```python
from build123d import *

# Parameters (mm, degrees)
SKETCH1_W           = 500
SKETCH1_H           = 50
BOSS_EXTRUDE1_DEPTH = 25
SKETCH2_R           = 10
CUT_EXTRUDE1_DEPTH  = 257.173769149
SKETCH4_R           = 25
BOSS_EXTRUDE2_DEPTH = 200
BOSS_EXTRUDE3_START = 200
SKETCH5_R           = 25
BOSS_EXTRUDE3_DEPTH = 200


with BuildPart() as part:
    # Sketch1 → Boss-Extrude1 (new, symmetric)
    with BuildSketch(Plane(origin=(0, 0, 0), x_dir=(1, 0, 0), z_dir=(0, 1, 0))):
        Rectangle(SKETCH1_W, SKETCH1_H)
    extrude(amount=BOSS_EXTRUDE1_DEPTH, both=True)

    # Sketch2 → Cut-Extrude1 (cut, through all)
    with BuildSketch(Plane(origin=(0, 25, 0), x_dir=(1, 0, 0), z_dir=(0, 1, 0))):
        with Locations(Location((200, 0, 0), (0, 0, 270))):
            Circle(SKETCH2_R)
        with Locations(Location((-200, 0, 0), (0, 0, 90))):
            Circle(SKETCH2_R)
    extrude(amount=-CUT_EXTRUDE1_DEPTH, mode=Mode.SUBTRACT)

    # Sketch4 → Boss-Extrude2 (add)
    with BuildSketch(Plane(origin=(250, 0, 0), x_dir=(0, 0, -1), z_dir=(1, 0, 0))):
        Circle(SKETCH4_R)
    extrude(amount=BOSS_EXTRUDE2_DEPTH)

    # Sketch5 → Boss-Extrude3 (add)
    with BuildSketch(Plane.ZY.offset(250).offset(BOSS_EXTRUDE3_START)):
        with Locations(Location((0, 0, 0), (0, 0, 180))):
            Circle(SKETCH5_R)
    extrude(amount=-BOSS_EXTRUDE3_DEPTH)


solid = part.part
```
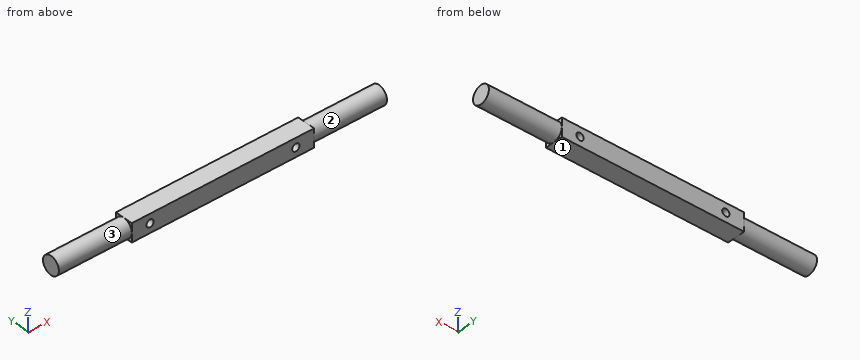
The model under review builds one solid part; all positions refer to its coordinate system, in mm. Face numbers are marked on the shaded views. A direction names the side the tool comes from. Coordinates: 2 decimals unless noted, no trailing zeros. Write each loop counter-clockwise with the first axis right and the second up, starting at its lowest first coordinate (ties: lowest second). Pieces come first, ordered by that corner, then holes. Notation, with made-up numbers: (66.25, 72) -> (70.25, 72) arc R28 cw to (70.25, 103) -> close; hole circle Ø4 at (68, 36). An arc over 180 degrees is marked (long way). One line per item, written item: value. Start each with the question number.
Q1. To check wall thickness, follow probe 1 along X at (y, z) = (2.5, 0); probe 2 along X at (y, z) = (2, 9); probe 3 along Z at (x, y) = (-200, 4). State the ranges of each line that lie inside material, in increasing order.
Q2. Add section A-A, the plane x = 200. Give the boundary of the cut face in (y, z).
Q3. Clearance check with flat-ended pins moving along their axes: P1, Ø12, axis at x = -284, z = -19, coming from the -Y side; P2, Ø3, axis at x = 260.5, y = -7.5, coming from the +Z side; P3, Ø5, axis at x = -310.5, z = 11, coming from the -Y side. State where each tip first meets the part, or that it passes through.
Q4. For the marked faces 1, 2 and 3, list the 3-axis set-ups (+Z, -Z, +X, -X, +Y, -Y) from which the entire face can be reached by the end or side of a thin tool; tool diameter is ignored.
Q5. Add section B-B, the plane y = -11. Give the boundary of the cut face in (x, z).
Q6. Add section C-C, the plane x = -366.5. Give the boundary of the cut face in (y, z).
Response:
1. probe 1: -450 to -210, -190 to 190, 210 to 450
1. probe 2: -450 to -204.36, -195.64 to 195.64, 204.36 to 450
1. probe 3: -25 to -10, 10 to 25
2. outline: (-25, -25) -> (25, -25) -> (25, -10) -> (-25, -10) -> close; (-25, 10) -> (25, 10) -> (25, 25) -> (-25, 25) -> close
3. P1: y = -21.35
3. P2: z = 24.27
3. P3: y = -23.51
4. face 1: -Z, +X, -X, +Y, -Y
4. face 2: +X
4. face 3: -X
5. outline: (-450, -22.45) -> (-250, -22.45) -> (-250, -25) -> (250, -25) -> (250, -22.45) -> (450, -22.45) -> (450, 22.45) -> (250, 22.45) -> (250, 25) -> (-250, 25) -> (-250, 22.45) -> (-450, 22.45) -> close; hole circle Ø20 at (-200, 0); hole circle Ø20 at (200, 0)
6. outline: circle Ø50 at (0, 0)
